For this review, take the finished solid that the model builds, in its own axes (mm). A direction names the side the tool comes from. Give positions to 0.01 mm unless a question says otherwise; leave off trailing zeros. Write each loop counter-clockwise with the first axis right and the second up, starting at its lowest first coordinate (ties: lowest second). Pieces come first, ordered by that corner, then holes. Notation, with made-up numbers: M -27.75,88 L -22.75,88 A25 ccw -22.75,112 Z; hole C 80,19.5 d4. An arc over 180 degrees is marked long. Write item = value, one per line.
```python
from build123d import *

# Parameters (mm, degrees)
F0_R     = 3.5
F0_R_2   = 3
F1_DEPTH = 17.016
F3_R     = 3.5
F3_R_2   = 1.143
F4_DEPTH = 16
F6_W     = 16
F6_H     = 9
F8_R     = 4.119335
F9_DEPTH = 10.16


with BuildPart() as f1:
    # F0 (on Top) → F1 (new body)
    with BuildSketch(Plane.XY):
        Circle(F0_R)
        Circle(F0_R_2, mode=Mode.SUBTRACT)
    extrude(amount=F1_DEPTH)

    # F3 (on offset) → F4 (join, through all)
    with BuildSketch(Plane.XY.offset(1.016)):
        Circle(F3_R)
        Circle(F3_R_2, mode=Mode.SUBTRACT)
    extrude(amount=F4_DEPTH)

    # F6 (on offset) → F7 section 0
    with BuildSketch(Plane.XY.offset(17.016), mode=Mode.PRIVATE) as f7_s0:
        Rectangle(F6_W, F6_H)
    loft([f7_s0.sketch, Vertex(0, 0, 1.016)], mode=Mode.SUBTRACT)

    # F8 (on offset) → F9 (cut)
    with BuildSketch(Plane.XY.offset(17.016)):
        Circle(F8_R)
    extrude(amount=-F9_DEPTH, mode=Mode.SUBTRACT)


solid = f1.part
```
1. Insertion check: P1, Ø2, axis at x = -1.5, z = 3, coming from the +Y side; P2, Ø3, axis at x = 0.5, y = 0, coming from the -Z side; P3, Ø1.5, axis at x = -1.5, z = 4, coming from the -Y side. Each pin has a flat end and moves straight along its axis. Give the tip position at first contact, or say it passes through.
Responses:
P1 = 3.46
P2 = 1.02
P3 = -3.42
2. The part is to be moulded in two halves that separate along X. For faces 4 (the face through (3, 1, 0)), 5 (the face through (2.158, -0.023, 5.333)), 6 (the face through (-2.158, 0.023, 5.333)), 7 (the face through (3.233, -1.341, 3.38)), say which applies: +X half, -X half, draft (parallel to the pull), parting line (faces both ways), or undercut.
Responses:
face_4 = draft
face_5 = undercut
face_6 = undercut
face_7 = parting line
3. Machinability: for faces 1 (the face through (1.3, 0, 1.016)), 2 (the face through (0.041, 1.334, 5.76)), 3 (the face through (1.09, 0.34, 2.57)), which of the approach directions +Z, -Z, +X, -X, +Y, -Y give a long, thin tool a straight path to every point of the face, cutting with its end or side? Answer none if there is none.
Responses:
face_1 = -Z
face_2 = +Z
face_3 = +Z, -Z
4. We need section C-C, the plane z = 4. Write out the cut boundary in (x, y).
Responses:
outline = C 0,0 d7; hole M -1.49,-0.84 L -0.78,-0.84 A1.14 ccw 0.78,-0.84 L 1.49,-0.84 L 1.49,0.84 L 0.78,0.84 A1.14 ccw -0.78,0.84 L -1.49,0.84 Z
5. We need section B-B, the plane y = 0. Write out the cut boundary in (x, z), then the cut area to 3 significant figures.
Responses:
outline = M -3.5,0 L -3,0 L -3,1.02 L -1.14,1.02 L -1.14,3.3 L -2.92,6.86 L -3.5,6.86 Z; M 1.14,1.02 L 3,1.02 L 3,0 L 3.5,0 L 3.5,6.86 L 2.92,6.86 L 1.14,3.3 Z
area = 22.2 mm2
6. We need section D-D, the plane y = 1.25. Write out the cut boundary in (x, z).
Responses:
outline = M -3.27,0 L -2.73,0 L -2.73,1.02 L 2.73,1.02 L 2.73,0 L 3.27,0 L 3.27,6.86 L 2.92,6.86 L 2.22,5.46 L -2.22,5.46 L -2.92,6.86 L -3.27,6.86 Z
7. We need section A-A, the plane x = 0. Write out the cut boundary in (y, z), then the cut area to 3 significant figures.
Responses:
outline = M -3.5,0 L -3,0 L -3,1.02 L -1.14,1.02 L -1.14,5.08 L -1.64,6.86 L -3.5,6.86 Z; M 1.14,1.02 L 3,1.02 L 3,0 L 3.5,0 L 3.5,6.86 L 1.64,6.86 L 1.14,5.08 Z
area = 27.7 mm2
8. For line 1 along X through (y, z) = (0, 1.85); line 2 along X through (y, z) = (0, 0.8), list the stretches that pass through material, from the lowest coordinate up. Write a range as from..to.
Responses:
line_1 = -3.5..-1.14, 1.14..3.5
line_2 = -3.5..-3, 3..3.5
